```python
from build123d import *

# Parameters (mm, degrees)
F0_R     = 6.35
F1_DEPTH = 3.175


# Not quite as in the source:
# - a feature names something its author has since deleted; it is built from what else it names


with BuildPart() as f1:
    # F0 (on Top) → F1 (new body)
    with BuildSketch(Plane.XY):
        with BuildLine():
            Line((50.546, -43.7890713215), (75.946, -43.7890713215))
            ThreePointArc((75.946, -43.7890713215), (80.4361280605, -41.929199382), (82.296, -37.4390713215))
            Line((82.296, -37.4390713215), (82.296, 38.7609286785))
            ThreePointArc((82.296, 38.7609286785), (80.4361280605, 43.251056739), (75.946, 45.1109286785))
            Line((75.946, 45.1109286785), (50.546, 45.1109286785))
            Line((50.546, 45.1109286785), (50.546, 42.5709286785))
            Line((50.546, 42.5709286785), (48.006, 42.5709286785))
            Line((48.006, 42.5709286785), (48.006, 45.1109286785))
            Line((48.006, 45.1109286785), (32.766, 45.1109286785))
            Line((32.766, 45.1109286785), (32.766, 42.5709286785))
            Line((32.766, 42.5709286785), (30.226, 42.5709286785))
            Line((30.226, 42.5709286785), (30.226, 45.1109286785))
            Line((30.226, 45.1109286785), (14.986, 45.1109286785))
            Line((14.986, 45.1109286785), (14.986, 42.5709286785))
            Line((14.986, 42.5709286785), (12.446, 42.5709286785))
            Line((12.446, 42.5709286785), (12.446, 45.1109286785))
            Line((12.446, 45.1109286785), (-38.354, 45.1109286785))
            Line((-38.354, 45.1109286785), (-38.354, -43.7890713215))
            Line((-38.354, -43.7890713215), (12.446, -43.7890713215))
            Line((12.446, -43.7890713215), (12.446, -41.2490713215))
            Line((12.446, -41.2490713215), (14.986, -41.2490713215))
            Line((14.986, -41.2490713215), (14.986, -43.7890713215))
            Line((14.986, -43.7890713215), (30.226, -43.7890713215))
            Line((30.226, -43.7890713215), (30.226, -41.2490713215))
            Line((30.226, -41.2490713215), (32.766, -41.2490713215))
            Line((32.766, -41.2490713215), (32.766, -43.7890713215))
            Line((32.766, -43.7890713215), (48.006, -43.7890713215))
            Line((48.006, -43.7890713215), (48.006, -41.2490713215))
            Line((48.006, -41.2490713215), (50.546, -41.2490713215))
            Line((50.546, -41.2490713215), (50.546, -43.7890713215))
        make_face()
        with Locations((-12.7, 0)):
            Circle(F0_R, mode=Mode.SUBTRACT)
        with BuildLine():
            Line((-82.804, -43.7890713215), (-38.354, -43.7890713215))
            Line((-38.354, -43.7890713215), (-38.354, 45.1109286785))
            Line((-38.354, 45.1109286785), (-82.804, 45.1109286785))
            Line((-82.804, 45.1109286785), (-82.804, 32.4109286785))
            ThreePointArc((-82.804, 32.4109286785), (-51.054, 0.6609286785), (-82.804, -31.0890713215))
            Line((-82.804, -31.0890713215), (-82.804, -43.7890713215))
        make_face()
    extrude(amount=F1_DEPTH)


solid = f1.part
```
Check sheet for the modelled part. Datum: model origin and axes. Units: mm. Round coordinates to 2 decimals unless told otherwise and drop trailing zeros. Order: outer loops, then holes, each group sorted by start corner. A loop starts at its lowest first (then second) coordinate and runs counter-clockwise, first axis right, second up. Notation, with made-up numbers: (12, 55.25) -> (23, 55.25) arc R21 cw to (23, 62.25) -> close; hole circle Ø7 at (-12.5, 49). An arc over 180 degrees is marked (long way). One line per item, written item: value. Start each with the question number.
Q1. Mould release check, pull along Y, two halves, no side actions. Record for faces 1 (the face through (40, 45.111, 2)), 2 (the face through (-6.643, 1.907, 1.565)), 3 (the face through (17, 1, 0)), 4 (the face through (-51.06, 1.36, 1.57)): pulls with the +Y half, pulls with the -Y half, needs draft (parallel to the pull), parting line crosses it, or undercut.
Q2. Cross-section at C-C (y = 0). Record the boundary of the cut face in (x, z) (3 decimals), and give its area (3 significant figures).
Q3. Cross-section at D-D (y = 14). Record the boundary of the cut face in (x, z) (3 decimals).
Q4. Cross-section at A-A (x = -12.7). Record the boundary of the cut face in (y, z) (3 decimals).
Q5. Gauge pin test, flat ends, axial feed: pin 1 Ø0.8 at (x, z) = (49.5, 1.5) entering from +Y; pin 2 Ø1.3 at (y, z) = (-42.5, 1.5) entering from +X; pin 3 Ø0.8 at (x, z) = (32, 1) entering from -Y. Record the tip position at first contact, or that the pin passes through.
Q6. Thickness scan on line 1 (Y direction, x = -12.7, z = 1.8); line 2 (Y direction, x = 48.5, z = 2.05); line 3 (Y direction, x = -64.5, z = 1.75). Record the ranges inside material, lowest first.
Completed:
1. face 1: pulls with the +Y half
1. face 2: undercut
1. face 3: needs draft
1. face 4: undercut
2. outline: (-51.061, 0) -> (-19.05, 0) -> (-19.05, 3.175) -> (-51.061, 3.175) -> close; (-6.35, 0) -> (82.296, 0) -> (82.296, 3.175) -> (-6.35, 3.175) -> close
2. area: 383 mm²
3. outline: (-53.992, 0) -> (82.296, 0) -> (82.296, 3.175) -> (-53.992, 3.175) -> close
4. outline: (-43.789, 0) -> (-6.35, 0) -> (-6.35, 3.175) -> (-43.789, 3.175) -> close; (6.35, 0) -> (45.111, 0) -> (45.111, 3.175) -> (6.35, 3.175) -> close
5. pin 1: stops at y = 42.57
5. pin 2: stops at x = 80.51
5. pin 3: stops at y = -41.25
6. line 1: y = -43.79 to -6.35, 6.35 to 45.11
6. line 2: y = -41.25 to 42.57
6. line 3: y = -43.79 to -25.28, 26.6 to 45.11
